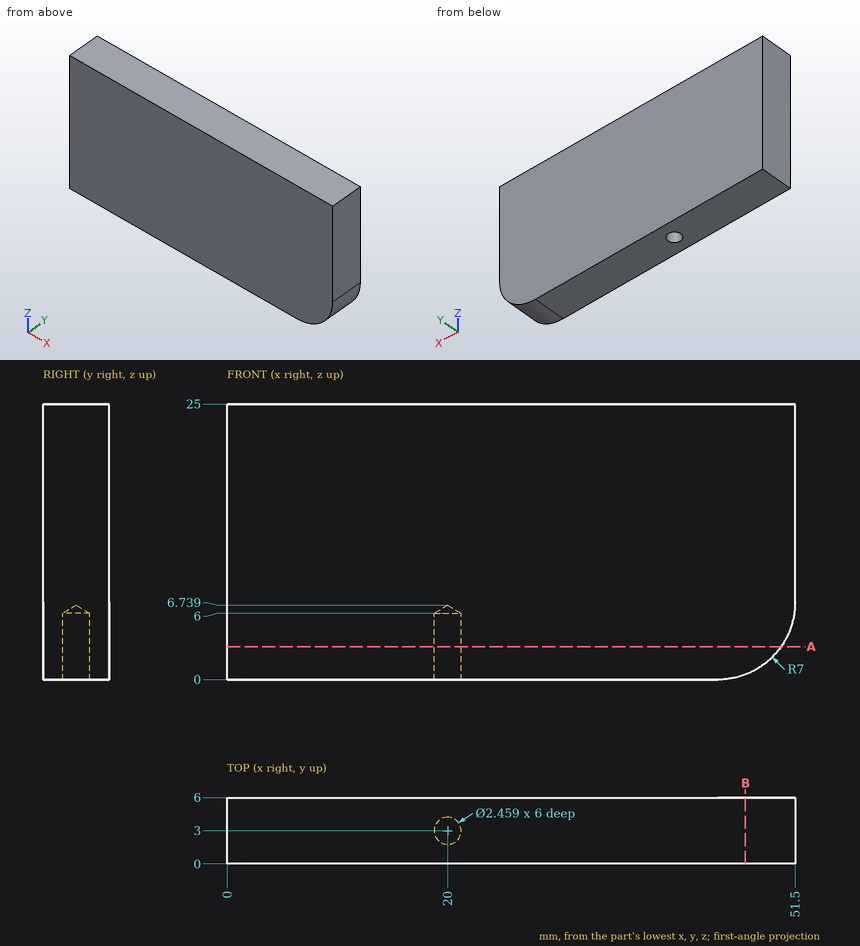
Check sheet for the drawn part. Datum: minimum x, y, z corner. Units: mm. Round coordinates to 2 decimals unless told otherwise and drop trailing zeros. Order: outer loops, then holes, each group sorted by start corner. A loop starts at its lowest first (then second) coordinate and runs counter-clockwise, first axis right, second up. Notation, with made-up numbers: (29, 14.5) -> (70, 14.5) arc R28 cw to (70, 52.5) -> close; hole circle Ø4 at (43.25, 70). An arc over 180 degrees is marked (long way). Return JSON: item names as keys, results as strings. Group by question number.
Q1. Section check B-B, the plane x = 47. Record the boundary of the cut face in (y, z).
Q2. Gauge pin test, flat ends, axial feed: pin 1 (3 mm diameter, centred on y = 5.5, z = 9.5, fed in from -X); pin 2 (2 mm diameter, centred on x = 20, y = 3, fed in from -Z). Record the tip position at first contact, or that the pin passes through.
Q3. Section check A-A, the plane z = 3. Record the boundary of the cut face in (x, y) (1 decimal), plus the area to 3 significant figures.
Q4. Material ranges on probe 1 along Y at (x, z) = (20, 4.15); probe 2 along X at (y, z) = (3, 4.8) (1 decimal); probe 3 along X at (y, z) = (3, 3.8) (1 decimal), recorded low to high. Write a range as from..to.
Numbers:
{
 "1": {"outline": "(0, 0.46) -> (6, 0.46) -> (6, 25) -> (0, 25) -> close"},
 "2": {"pin 1": "x = 0", "pin 2": "z = 6.14"},
 "3": {"outline": "(0, 0) -> (50.2, 0) -> (50.2, 6) -> (0, 6) -> close; hole circle Ø2.5 at (20, 3)", "area": "297 mm^2"},
 "4": {"probe 1": "0..1.77, 4.23..6", "probe 2": "0..18.8, 21.2..51.1", "probe 3": "0..18.8, 21.2..50.7"}
}
